Build history of the part. All positions in model axes, mm. Round coordinates to 2 decimals unless told otherwise and drop trailing zeros. Loops run counter-clockwise (first coordinate to the right, second up) from the corner with the lowest first, then second, coordinate; pieces in that order, holes last. Notation, with made-up numbers: (36, 72) -> (55, 72) arc R27 ccw to (55, 98) -> close; hole circle Ø9 at (-15, -35). An arc over 180 degrees is marked (long way). Put each result on its own line as item: value. Start each with the question number.
Item 1: Cut at B-B, the plane x = 0. List the corners of the cut face in (y, z).
Item 2: Cut at A-A, the plane y = 0. List the corners of the cut face in (x, z), plus the area to 3 significant figures.
Item 3: Flat gauge pins, fed straight in: pin 1 Ø2.5 at (x, y) = (0, -35) entering from +Z; pin 2 Ø1.5 at (x, z) = (17, 1.5) entering from +Y; pin 3 Ø1.5 at (x, z) = (14, 2) entering from -Y; pin 4 Ø1 at (y, z) = (18, 0.5) entering from +X. Where does each tip first touch, or does it go through?
Item 4: Drill centre lines: probe 1 along Y at (x, z) = (0, 2); probe 2 along Y at (x, z) = (20, 2.2); probe 3 along X at (y, z) = (-21.5, 1.45). Where is each one in solid material? Low to high. Write a range as [from, to].
Item 5: Cut at C-C, the plane y = 15. List the corners of the cut face in (x, z), plus the area to 3 significant figures.
Item 6: Cut at D-D, the plane z = 0.8. Count the separate pieces of the cut face and the enclosed holes in it, plus the area to 3 significant figures.
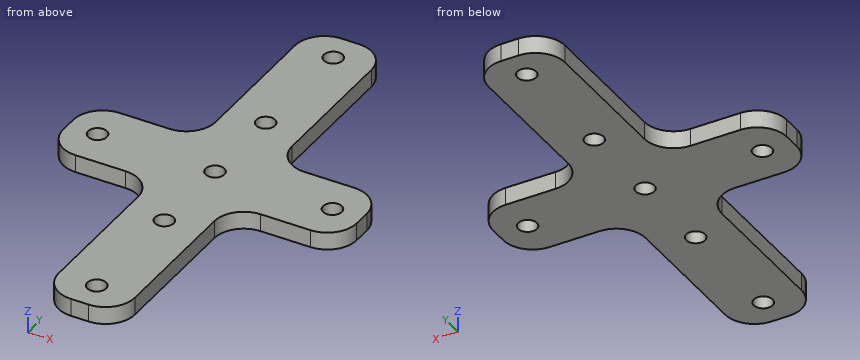
```python
from build123d import *

# Parameters (mm, degrees)
SKETCH_1_R      = 1.6
EXTRUDE_1_DEPTH = 3
FILLET_1_R      = 5


with BuildPart() as part:
    # 草图1 → 凸台-拉伸1 (new body)
    with BuildSketch(Plane.XY):
        Polygon((-6.5, 6.5), (-25, 6.5), (-25, -6.5), (25, -6.5), (25, 6.5), (6.5, 6.5), (6.5, 40), (-6.5, 40), align=None)
        with Locations((0, 35)):
            Circle(SKETCH_1_R, mode=Mode.SUBTRACT)
        with Locations((0, 15)):
            Circle(SKETCH_1_R, mode=Mode.SUBTRACT)
        Circle(SKETCH_1_R, mode=Mode.SUBTRACT)
        with Locations((20, 0)):
            Circle(SKETCH_1_R, mode=Mode.SUBTRACT)
        with Locations((-20, 0)):
            Circle(SKETCH_1_R, mode=Mode.SUBTRACT)
    extrude(amount=EXTRUDE_1_DEPTH)

    # 圆角1
    fillet_1_edges = [part.edges().sort_by_distance(p)[0] for p in [
        (-6.5, 40, 1.5),
        (6.5, 40, 1.5),
        (6.5, 6.5, 1.5),
        (25, 6.5, 1.5),
        (25, -6.5, 1.5),
        (-25, -6.5, 1.5),
        (-25, 6.5, 1.5),
        (-6.5, 6.5, 1.5),
    ]]
    fillet(fillet_1_edges, radius=FILLET_1_R)

    # 镜向1: part across plane


with BuildPart() as part_1:
    add(part.part)
    add(part.part.mirror(Plane.ZX))


solid = part_1.part
```
Reply:
1. outline: (-40, 0) -> (-36.6, 0) -> (-36.6, 3) -> (-40, 3) -> close; (-33.4, 0) -> (-16.6, 0) -> (-16.6, 3) -> (-33.4, 3) -> close; (-13.4, 0) -> (-1.6, 0) -> (-1.6, 3) -> (-13.4, 3) -> close; (1.6, 0) -> (13.4, 0) -> (13.4, 3) -> (1.6, 3) -> close; (16.6, 0) -> (33.4, 0) -> (33.4, 3) -> (16.6, 3) -> close; (36.6, 0) -> (40, 0) -> (40, 3) -> (36.6, 3) -> close
2. outline: (-25, 0) -> (-21.6, 0) -> (-21.6, 3) -> (-25, 3) -> close; (-18.4, 0) -> (-1.6, 0) -> (-1.6, 3) -> (-18.4, 3) -> close; (1.6, 0) -> (18.4, 0) -> (18.4, 3) -> (1.6, 3) -> close; (21.6, 0) -> (25, 0) -> (25, 3) -> (21.6, 3) -> close
2. area: 121 mm^2
3. pin 1: passes through
3. pin 2: stops at y = 6.5
3. pin 3: stops at y = -6.5
3. pin 4: stops at x = 6.5
4. probe 1: y = [-40, -36.6], [-33.4, -16.6], [-13.4, -1.6], [1.6, 13.4], [16.6, 33.4], [36.6, 40]
4. probe 2: y = [-6.5, -1.6], [1.6, 6.5]
4. probe 3: x = [-6.5, 6.5]
5. outline: (-6.5, 0) -> (-1.6, 0) -> (-1.6, 3) -> (-6.5, 3) -> close; (1.6, 0) -> (6.5, 0) -> (6.5, 3) -> (1.6, 3) -> close
5. area: 29.4 mm^2
6. separate pieces: 1
6. enclosed holes: 7
6. area: 1,440 mm^2
